The model under review builds one solid part; all positions refer to its coordinate system, in mm. Round coordinates to 2 decimals unless told otherwise and drop trailing zeros. Order: outer loops, then holes, each group sorted by start corner. A loop starts at its lowest first (then second) coordinate and runs counter-clockwise, first axis right, second up. Notation, with made-up numbers: (87.5, 51.5) -> (111.5, 51.5) arc R5 ccw to (111.5, 59.5) -> close; hole circle Ø2 at (64.5, 46). An arc over 180 degrees is marked (long way). Put each result on its own line as item: value. Start each with the question number.
from build123d import *

# Parameters (mm, degrees)
SKETCH1_W                = 63.9
SKETCH1_H                = 24
BOSS_EXTRUDE1_DEPTH      = 7.7
F_5_16_18_TAPPED_HOLE1_D = 6.5278
CUT_EXTRUDE1_DEPTH       = 69.69133861


with BuildPart() as part:
    # Sketch1 → Boss-Extrude1 (new body)
    with BuildSketch(Plane.XY):
        with Locations((31.95, 12)):
            Rectangle(SKETCH1_W, SKETCH1_H)
    extrude(amount=BOSS_EXTRUDE1_DEPTH)

    # 5/16-18 Tapped Hole1 (through all)
    with Locations(Plane(origin=(8.1375, 12, 7.7), x_dir=(1, 0, 0), z_dir=(0, 0, 1))):
        with Locations((0, 0), (47.625, 0)):
            Hole(F_5_16_18_TAPPED_HOLE1_D / 2)

    # Sketch4 → Cut-Extrude1 (cut, through all)
    with BuildSketch(Plane.XY.offset(7.7)):
        with BuildLine():
            ThreePointArc((0, 18.867585454), (10.39806648, 22.698962504), (21.402908053, 24))
            Line((21.402908053, 24), (0, 24))
            Line((0, 24), (0, 18.867585454))
        make_face()
        with BuildLine():
            Line((0, 0), (21.402908053, 0))
            ThreePointArc((21.402908053, 0), (10.39806648, 1.301037496), (0, 5.132414546))
            Line((0, 5.132414546), (0, 0))
        make_face()
        with BuildLine():
            Line((63.9, 0), (63.9, 5.132414546))
            ThreePointArc((63.9, 5.132414546), (53.50193352, 1.301037496), (42.497091947, 0))
            Line((42.497091947, 0), (63.9, 0))
        make_face()
        with BuildLine():
            Line((63.9, 18.867585454), (63.9, 24))
            Line((63.9, 24), (42.497091947, 24))
            ThreePointArc((42.497091947, 24), (53.50193352, 22.698962504), (63.9, 18.867585454))
        make_face()
    extrude(amount=-CUT_EXTRUDE1_DEPTH, mode=Mode.SUBTRACT)


solid = part.part
Q1. Take a section at A-A on y = 12. Give the boundary of the cut face in (x, z), and give its area (3 significant figures).
Q2. Draft analysis for pull direction X (two halves, no side actions). For faces 1 (the face through (53.351, 22.735, 3.904)), 2 (the face through (32, 12, 7.7)), 3 (the face through (10.549, 1.265, 3.904)), 4 (the face through (10.728, 10.014, 3.796)), state which applies: +X half, -X half, draft (parallel to the pull), parting line (faces both ways), or undercut.
Q3. Wall thickness on probe 1 along Y at (x, z) = (6, 7); probe 2 along X at (y, z) = (20, 1.5); probe 3 along Y at (x, z) = (58, 7): over which ranges is each line inside the solid? List them lowest first. Write a range as [from, to].
Q4. Take a section at D-D on y = 9.5. Give the boundary of the cut face in (x, z).
Q5. Clearance check with flat-ended pins moving along their axes: pin 1 Ø1 at (y, z) = (21, 6) entering from +X; pin 2 Ø1 at (x, z) = (19, 3.5) entering from -Y. State where each tip first meets the part, or that it passes through.
Q6. Take a section at B-B on z = 0.75. Give the boundary of the cut face in (x, y).
Q7. Take a section at C-C on x = 54. Give the boundary of the cut face in (y, z).
Calculated:
1. outline: (0, 0) -> (4.87, 0) -> (4.87, 7.7) -> (0, 7.7) -> close; (11.4, 0) -> (52.5, 0) -> (52.5, 7.7) -> (11.4, 7.7) -> close; (59.03, 0) -> (63.9, 0) -> (63.9, 7.7) -> (59.03, 7.7) -> close
1. area: 392 mm²
2. face 1: +X half
2. face 2: draft
2. face 3: -X half
2. face 4: undercut
3. probe 1: y = [2.58, 9.53], [14.47, 21.42]
3. probe 2: x = [2.39, 61.51]
3. probe 3: y = [2.62, 9.62], [14.38, 21.38]
4. outline: (0, 0) -> (6.04, 0) -> (6.04, 7.7) -> (0, 7.7) -> close; (10.24, 0) -> (53.66, 0) -> (53.66, 7.7) -> (10.24, 7.7) -> close; (57.86, 0) -> (63.9, 0) -> (63.9, 7.7) -> (57.86, 7.7) -> close
5. pin 1: stops at x = 60.33
5. pin 2: stops at y = 0.04
6. outline: (0, 5.13) arc R47.19 ccw to (21.4, 0) -> (42.5, 0) arc R47.19 ccw to (63.9, 5.13) -> (63.9, 18.87) arc R47.19 ccw to (42.5, 24) -> (21.4, 24) arc R47.19 ccw to (0, 18.87) -> close; hole circle Ø6.53 at (8.14, 12); hole circle Ø6.53 at (55.76, 12)
7. outline: (1.42, 0) -> (9.25, 0) -> (9.25, 7.7) -> (1.42, 7.7) -> close; (14.75, 0) -> (22.58, 0) -> (22.58, 7.7) -> (14.75, 7.7) -> close
